Autodesk Inventor part; units mm, degrees
ref_plane "YZ Plane" through (0, 0, 0) normal (1, 0, 0) x (0, 1, 0)
ref_plane "XZ Plane" through (0, 0, 0) normal (0, 1, 0) x (-1, 0, 0)
ref_plane "XY Plane" through (0, 0, 0) normal (0, 0, 1) x (1, 0, 0)
sketch "Sketch1" plane through (0, 0, 0) normal (0, 1, 0) x (-1, 0, 0)
  line L0 (405.5305, 409.815) -> (465.5305, 409.815) construction
  line L1 (405.5305, 379.815) -> (405.5305, 409.815) construction
  line L2 (460.5305, 404.815) -> (410.5305, 404.815)
  line L3 (410.5305, 404.815) -> (410.5305, 379.815)
  line L4 (460.5305, 386.815) -> (470.5305, 386.815)
  line L5 (470.5305, 414.815) -> (465.2753, 414.815)
  line L6 (400.5305, 414.815) -> (400.5305, 409.5598) construction
  line L7 (465.5305, 409.815) -> (465.5305, 386.815) construction
  line L8 (460.5305, 386.815) -> (460.5305, 404.815)
  line L9 (470.5305, 386.815) -> (470.5305, 409.5598)
  line L10 (405.5305, 409.815) -> (400.5305, 414.815) construction
  line L11 (400.5305, 379.815) -> (470.5305, 379.815) construction
  line L12 (465.5305, 409.815) -> (470.5305, 414.815) construction
  arc A0 (405.7856, 414.815) -> (400.5305, 409.5598) centre (402.1112, 413.2342) ccw
  arc A1 (404.9397, 410.4058) -> (405.7856, 414.815) centre (402.1112, 413.2342) ccw construction
  line L13 (400.5305, 409.5598) -> (400.5305, 379.815)
  arc A2 (400.5305, 409.5598) -> (404.9397, 410.4058) centre (402.1112, 413.2342) ccw construction
  line L14 (405.7856, 414.815) -> (400.5305, 414.815) construction
  circle A3 centre (402.1112, 413.2342) radius 1.3
  line L15 (435.5305, 414.815) -> (435.5305, 379.815) construction
  arc A4 (465.2753, 414.815) -> (470.5305, 409.5598) centre (468.9497, 413.2342) ccw construction
  arc A5 (470.5305, 409.5598) -> (465.2753, 414.815) centre (468.9497, 413.2342) ccw
  line L16 (470.5305, 409.5598) -> (470.5305, 414.815) construction
  line L17 (465.2753, 414.815) -> (405.7856, 414.815)
  circle A6 centre (468.9497, 413.2342) radius 1.3
  line L18 (460.5305, 372.815) -> (460.5305, 354.815)
  line L19 (465.5305, 349.815) -> (465.5305, 372.815) construction
  line L20 (460.5305, 372.815) -> (470.5305, 372.815)
  line L21 (470.5305, 372.815) -> (470.5305, 350.0701)
  arc A7 (470.5305, 350.0701) -> (465.2753, 344.815) centre (468.9497, 346.3957) ccw construction
  line L22 (470.5305, 344.815) -> (465.2753, 344.815) construction
  line L23 (465.5305, 349.815) -> (470.5305, 344.815) construction
  line L24 (470.5305, 350.0701) -> (470.5305, 344.815) construction
  arc A8 (465.2753, 344.815) -> (470.5305, 350.0701) centre (468.9497, 346.3957) ccw
  circle A9 centre (468.9497, 346.3957) radius 1.3
  line L25 (400.5305, 344.815) -> (400.5305, 350.0701) construction
  circle A10 centre (402.1112, 346.3957) radius 1.3
  line L26 (405.5305, 349.815) -> (400.5305, 344.815) construction
  line L27 (405.7856, 344.815) -> (400.5305, 344.815) construction
  arc A11 (400.5305, 350.0701) -> (405.7856, 344.815) centre (402.1112, 346.3957) ccw
  line L28 (435.5305, 344.815) -> (435.5305, 379.815) construction
  line L29 (405.5305, 349.815) -> (465.5305, 349.815) construction
  line L30 (460.5305, 354.815) -> (410.5305, 354.815)
  arc A12 (405.7856, 344.815) -> (404.9397, 349.2242) centre (402.1112, 346.3957) ccw construction
  line L31 (410.5305, 354.815) -> (410.5305, 379.815)
  line L32 (405.5305, 379.815) -> (405.5305, 349.815)
  line L33 (400.5305, 350.0701) -> (400.5305, 379.815)
  arc A13 (404.9397, 349.2242) -> (400.5305, 350.0701) centre (402.1112, 346.3957) ccw construction
  circle A14 centre (415.5305, 340.824) radius 1.3
  arc A15 (412.0305, 340.824) -> (419.0305, 340.824) centre (415.5305, 340.824) ccw
  line L34 (412.0305, 340.824) -> (412.0305, 344.815)
  line L35 (419.0305, 340.824) -> (419.0305, 344.815)
  line L36 (452.0305, 340.824) -> (452.0305, 344.815)
  circle A16 centre (455.5305, 340.824) radius 1.3
  arc A17 (452.0305, 340.824) -> (459.0305, 340.824) centre (455.5305, 340.824) ccw
  line L37 (459.0305, 340.824) -> (459.0305, 344.815)
  line L38 (412.0305, 344.815) -> (405.7856, 344.815)
  line L39 (465.2753, 344.815) -> (459.0305, 344.815)
  line L40 (452.0305, 344.815) -> (419.0305, 344.815)
  point P0 (0, 0)
  point P1 (403.0305, 412.315)
  point P2 (468.0305, 412.315)
  point P3 (468.0305, 347.315)
  point P4 (403.0305, 347.315)
  dimension "d0" = 23
  dimension "d1" = 5
  dimension "d2" = 8
  dimension "d3" = 2.6
  dimension "d4" = 8
  dimension "d5" = 2.6
  dimension "d6" = 2.6
  dimension "d7" = 20
  dimension "d8" = 35
  dimension "d9" = 7
extrude "Extrusion1" add sketch "Sketch1" along normal blind 3.175
properties part number "trellisCaptiveTop"
The model under review builds one solid part; all positions refer to its coordinate system, in mm. A direction names the side the tool comes from. Give positions to 0.01 mm unless a question says otherwise; leave off trailing zeros. Order: outer loops, then holes, each group sorted by start corner. A loop starts at its lowest first (then second) coordinate and runs counter-clockwise, first axis right, second up. Notation, with made-up numbers: (87, -18.75) - (94, -18.75) arc R21 cw to (94, -11.75) - close; hole circle Ø6 at (-18.5, 38.25). An arc over 180 degrees is marked (long way). Use CSV: the item, a comma, the result in double quotes. Start each with the question number.
Q1. We need section A-A, the plane z = 403. Write out the cut boundary in (x, y) (1 decimal).
Q2. Tool access review of faces 1 (the flat face through (-459.03, 2, 343)), 2 (the flat face through (-465, 2, 372.815)), 3 (the flat face through (-410, 3.175, 378)), 4 (the flat face through (-460.53, 2, 364)): name each direction out of +Z, -Z, +X, -X, +Y, -Y from which nothing blocks a thin tool from reaching the whole face with its end or side.
Q3. We need section B-B, the plane x = -424.5. Write out the cut boundary in (y, z) (3 decimals).
Q4. We need section D-D, the plane z = 375.5. Write out the cut boundary in (x, y) (1 decimal), and give its area (4 significant figures).
Q5. We need section C-C, the plane y = 1.8. State how many separate pieces and enclosed holes the cut face has, and give its area (3 significant figures).
Q6. Clearance check with flat-ended pins moving along their axes: pin 1 Ø1.5 at (x, y) = (-444.5, 1.5) entering from +Z (3 decimals); pin 2 Ø1 at (y, z) = (1, 364.5) entering from +X; pin 3 Ø1.6 at (y, z) = (1, 342.5) entering from +X. State where each tip first meets the part, or that it passes through.
Q7. The part is to be moulded in two halves that separate along Z. For faces 5 (the flat face through (-452.03, 2, 343)), 6 (the cylindrical face through (-399.207, 1.565, 415.984)), 7 (the cylindrical face through (-415.607, 1.565, 337.325)), 8 (the flat face through (-436, 2, 414.815)), say which applies: +Z half, -Z half, draft (parallel to the pull), parting line (faces both ways), or undercut.
Q8. To check wall thickness, follow line 1 along X through (y, z) = (2.55, 390); line 2 along Z through (x, y) = (-465, 1.5) (3 decimals); line 3 along Z through (x, y) = (-446.5, 0.3) (3 decimals). State the ranges of each line that lie inside material, in increasing order. Write a range as [from, to].
Outcome:
1,outline,"(-470.5, 0) - (-460.5, 0) - (-460.5, 3.2) - (-470.5, 3.2) - close; (-410.5, 0) - (-400.5, 0) - (-400.5, 3.2) - (-410.5, 3.2) - close"
2,face 1,"-Z, +Y, -Y"
2,face 2,"-X, +Y, -Y"
2,face 3,"+Z, -Z, +X, -X, +Y"
2,face 4,"+Y, -Y"
3,outline,"(0, 344.815) - (3.175, 344.815) - (3.175, 354.815) - (0, 354.815) - close; (0, 404.815) - (3.175, 404.815) - (3.175, 414.815) - (0, 414.815) - close"
4,outline,"(-410.5, 0) - (-400.5, 0) - (-400.5, 3.2) - (-410.5, 3.2) - close"
4,area,"31.75 mm^2"
5,separate pieces,"1"
5,enclosed holes,"6"
5,area,"2,410 mm^2"
6,pin 1,"stops at z = 414.815"
6,pin 2,"stops at x = -400.53"
6,pin 3,"stops at x = -399.58"
7,face 5,"draft"
7,face 6,"undercut"
7,face 7,"-Z half"
7,face 8,"+Z half"
8,line 1,"x = [-470.53, -460.53], [-410.53, -400.53]"
8,line 2,"z = [344.815, 372.815], [386.815, 414.815]"
8,line 3,"z = [344.815, 354.815], [404.815, 414.815]"
